Autodesk Inventor part; units mm, degrees
ref_plane "YZ Plane" through (0, 0, 0) normal (1, 0, 0) x (0, 1, 0)
ref_plane "XZ Plane" through (0, 0, 0) normal (0, 1, 0) x (-1, 0, 0)
ref_plane "XY Plane" through (0, 0, 0) normal (0, 0, 1) x (1, 0, 0)
sketch "Sketch1" plane through (0, 0, 0) normal (0, 0, 1) x (1, 0, 0)
  line L0 (13.75, -9.25) -> (-13.75, -9.25)
  line L1 (-13.75, -9.25) -> (-13.75, 9.25)
  line L2 (-13.75, 9.25) -> (13.75, 9.25)
  line L3 (13.75, 9.25) -> (13.75, -9.25)
  line L4 (13.75, -9.25) -> (-13.75, 9.25) construction
  line L5 (-13.75, -9.25) -> (13.75, 9.25) construction
  point P0 (0, 0)
  dimension "d0" = 27.5
  dimension "d1" = 18.5
extrude "Extrusion1" add sketch "Sketch1" along normal blind 4.7625
sketch "Sketch2" plane through (0, 0, 4.7625) normal (0, 0, 1) x (1, 0, 0)
  line L0 (10, -5.5) -> (-10, -5.5) construction
  line L1 (-10, -5.5) -> (-10, 5.5) construction
  line L2 (-10, 5.5) -> (10, 5.5) construction
  line L3 (10, 5.5) -> (10, -5.5) construction
  line L4 (10, -5.5) -> (-10, 5.5) construction
  line L5 (-10, -5.5) -> (10, 5.5) construction
  point P0 (0, 0)
  dimension "d4" = 20
  dimension "d5" = 11
hole "Hole1" at (-10, 5.5, 4.7625) at (10, 5.5, 4.7625) at (10, -5.5, 4.7625) at (-10, -5.5, 4.7625) direction (0, 0, -1) diameter 3.3 end through all
sketch "Sketch3" plane through (0, 0, 4.7625) normal (0, 0, 1) x (1, 0, 0)
  point P0 (0, 0)
hole "Hole2" at (0, 0, 4.7625) direction (0, 0, -1) diameter 6.5 end through all
fillet "Fillet1" radius 2 4 edges at (-13.75, 9.25, 2.3813) (-13.75, -9.25, 2.3813) (13.75, -9.25, 2.3813) (13.75, 9.25, 2.3813)
properties part number "Printhead Belt Retainer Top Spacer" material "Aluminum 6061"
Source: CAD feature listing. Evaluate the final solid. Frame: model axes, mm. Give positions to 0.01 mm unless a question says otherwise; leave off trailing zeros. Loops run counter-clockwise (first coordinate to the right, second up) from the corner with the lowest first, then second, coordinate; pieces in that order, holes last. Notation, with made-up numbers: (30, 47) -> (68, 47) arc R15 cw to (68, 64) -> close; hole circle Ø2 at (5, 58.5). An arc over 180 degrees is marked (long way). Put each result on its own line as item: value. Start each with the question number.
1) Cut plane B-B (z = 2.1). Return loops of the section in (x, y), then the cut area to 3 significant figures.
2) Cut plane C-C (x = 10). Return loops of the section in (y, z), then the cut area to 3 significant figures.
3) Contact query for a flat-ended pin moving along its axis: P1, Ø4, axis at x = 10, y = 5.5, coming from the -Z side. Output: stop coordinate, or through.
4) Cut plane A-A (y = 5.5). Return loops of the section in (x, z).
5) Draft query along Y for faces 1 (the face through (-13.15, 8.68, 2.41)), 2 (the face through (1.978, 2.579, 2.348)), 3 (the face through (0, -9.25, 2)). Return one class per face: released by +Y, released by -Y, zero draft, split by the parting line, or undercut.
6) Cut plane D-D (x = 1.25). Return loops of the section in (y, z).
7) Material intervals for probe 1 along Y at (x, z) = (-10, 3.2); probe 2 along X at (y, z) = (5.5, 3.8); probe 3 along Y at (x, z) = (-8.75, 0.95), sorted ascending.
Results are:
1. outline: (-13.75, -7.25) arc R2 ccw to (-11.75, -9.25) -> (11.75, -9.25) arc R2 ccw to (13.75, -7.25) -> (13.75, 7.25) arc R2 ccw to (11.75, 9.25) -> (-11.75, 9.25) arc R2 ccw to (-13.75, 7.25) -> close; hole circle Ø3.3 at (-10, -5.5); hole circle Ø3.3 at (-10, 5.5); hole circle Ø6.5 at (0, 0); hole circle Ø3.3 at (10, -5.5); hole circle Ø3.3 at (10, 5.5)
1. area: 438 mm2
2. outline: (-9.25, 0) -> (-7.15, 0) -> (-7.15, 4.76) -> (-9.25, 4.76) -> close; (-3.85, 0) -> (3.85, 0) -> (3.85, 4.76) -> (-3.85, 4.76) -> close; (7.15, 0) -> (9.25, 0) -> (9.25, 4.76) -> (7.15, 4.76) -> close
2. area: 56.7 mm2
3. P1: stops at z = 0
4. outline: (-13.75, 0) -> (-11.65, 0) -> (-11.65, 4.76) -> (-13.75, 4.76) -> close; (-8.35, 0) -> (8.35, 0) -> (8.35, 4.76) -> (-8.35, 4.76) -> close; (11.65, 0) -> (13.75, 0) -> (13.75, 4.76) -> (11.65, 4.76) -> close
5. face 1: released by +Y
5. face 2: undercut
5. face 3: released by -Y
6. outline: (-9.25, 0) -> (-3, 0) -> (-3, 4.76) -> (-9.25, 4.76) -> close; (3, 0) -> (9.25, 0) -> (9.25, 4.76) -> (3, 4.76) -> close
7. probe 1: y = -9.25 to -7.15, -3.85 to 3.85, 7.15 to 9.25
7. probe 2: x = -13.75 to -11.65, -8.35 to 8.35, 11.65 to 13.75
7. probe 3: y = -9.25 to -6.58, -4.42 to 4.42, 6.58 to 9.25
